Source: CAD feature listing. Evaluate the final solid. Frame: model axes, mm. Round coordinates to 2 decimals unless told otherwise and drop trailing zeros. Write each loop counter-clockwise with the first axis right and the second up, starting at its lowest first coordinate (ties: lowest second). Pieces come first, ordered by that corner, then holes.
from build123d import *

# Parameters (mm, degrees)
F0_R     = 3.776883
F0_W     = 13.310812
F0_H     = 5.56634
F1_DEPTH = 7.62


with BuildPart() as f1:
    # F0 (on Top) → F1 (new body)
    with BuildSketch(Plane.XY):
        Polygon((-125.915021, 62.309951), (-125.915021, -22.304947), (18.851278, -22.304947), (18.851278, -6.763435), (26.622031, -6.763435), (26.622031, -22.017142), (118.144266, -22.304947), (118.144266, 41.58793), (111.525701, 41.608743), (111.501263, 31.801704), (26.622031, 32.068619), (26.622031, 16.836636), (18.851278, 16.836636), (18.851278, 31.801704), (-47.428191, 32.010129), (-47.428191, 41.608743), (-55.215195, 41.608743), (-55.215195, 32.034616), (-93.54344, 32.034616), (-93.54344, 62.309951), align=None)
        with Locations((22.773762, 5.0366)):
            Circle(F0_R, mode=Mode.SUBTRACT)
        with Locations((-114.20754, 56.850752)):
            Rectangle(F0_W, F0_H, mode=Mode.SUBTRACT)
    extrude(amount=F1_DEPTH)


solid = f1.part
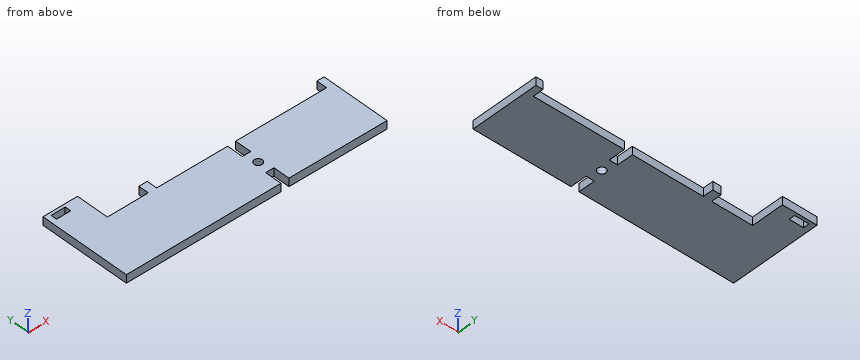
1) Section query A-A on y = 29. Return the cut outline in (x, z), then the cut area to 3 significant figures.
Taken from the geometry:
outline: (-125.92, 0) - (18.85, 0) - (18.85, 7.62) - (-125.92, 7.62) - close; (26.62, 0) - (118.14, 0) - (118.14, 7.62) - (26.62, 7.62) - close
area: 1,800 mm2
2) Material intervals for line 1 (X direction, y = 36, z = 4); line 2 (Y direction, x = -109, z = 2.75); line 3 (X direction, y = -13, z = 5.75), sorted ascending.
Taken from the geometry:
line 1: x = -125.92 to -93.54, -55.22 to -47.43, 111.51 to 118.14
line 2: y = -22.3 to 54.07, 59.63 to 62.31
line 3: x = -125.92 to 18.85, 26.62 to 118.14
3) Section query D-D on x = 69. Return the cut outline in (y, z).
Taken from the geometry:
outline: (-22.15, 0) - (31.94, 0) - (31.94, 7.62) - (-22.15, 7.62) - close
4) Contact query for flat-ended pins moving along their axis: P1, Ø4, axis at y = 42, z = 2.5, coming from the +X side; P2, Ø4, axis at x = -78, z = 3, coming from the +Y side; P3, Ø2.5, axis at x = 23, z = 2.5, coming from the +Y side; P4, Ø2.5, axis at x = 21, z = 3, coming from the -Y side. Output: stop coordinate, or through.
Taken from the geometry:
P1: stops at x = 118.14
P2: stops at y = 32.03
P3: stops at y = 16.84
P4: stops at y = -6.76
5) Section query C-C on y = 38.5. Return the cut outline in (x, z), then the cut area to 4 significant figures.
Taken from the geometry:
outline: (-125.92, 0) - (-93.54, 0) - (-93.54, 7.62) - (-125.92, 7.62) - close; (-55.22, 0) - (-47.43, 0) - (-47.43, 7.62) - (-55.22, 7.62) - close; (111.52, 0) - (118.14, 0) - (118.14, 7.62) - (111.52, 7.62) - close
area: 356.5 mm2
6) Section query B-B on z = 2.5. Return the cut outline in (x, y).
Taken from the geometry:
outline: (-125.92, -22.3) - (18.85, -22.3) - (18.85, -6.76) - (26.62, -6.76) - (26.62, -22.02) - (118.14, -22.3) - (118.14, 41.59) - (111.53, 41.61) - (111.5, 31.8) - (26.62, 32.07) - (26.62, 16.84) - (18.85, 16.84) - (18.85, 31.8) - (-47.43, 32.01) - (-47.43, 41.61) - (-55.22, 41.61) - (-55.22, 32.03) - (-93.54, 32.03) - (-93.54, 62.31) - (-125.92, 62.31) - close; hole (-120.86, 54.07) - (-107.55, 54.07) - (-107.55, 59.63) - (-120.86, 59.63) - close; hole circle Ø7.55 at (22.77, 5.04)
